Build history of the part. All positions in model axes, mm. A direction names the side the tool comes from. Give positions to 0.01 mm unless a question says otherwise; leave off trailing zeros. Order: outer loops, then holes, each group sorted by start corner. A loop starts at its lowest first (then second) coordinate and runs counter-clockwise, first axis right, second up. Notation, with made-up numbers: (48, 13.5) - (102, 13.5) arc R20 cw to (102, 31.5) - close; hole circle Ø9 at (63, 25.5). An arc over 180 degrees is marked (long way). Use a Markdown table: item, result. Add a question column.
(1) Mould opens along Y. For faces 6 (the face through (18, 2, 2.54)), 7 (the face through (31.772, 12.75, 1.288)), 8 (the face through (27.292, 8.809, 6.332)) say: +Y half, -Y half, draft (parallel to the pull), parting line (faces both ways), or undercut.
(2) Slice it at D-D (z = 11.5). Write the cut outline in (x, y).
(3) Slice it at B-B (y = 10.5). Write the cut outline in (x, z).
(4) Flat gauge pins, fed straight in: pin 1 (1.3 mm diameter, centred on x = 23, z = 4.5, fed in from -Y); pin 2 (5 mm diameter, centred on x = 11, y = 7.5, fed in from +Z); pin 3 (3 mm diameter, centred on x = 11.5, y = 17, fed in from +Z). Where does each tip first touch, or does it go through?
(5) Which spindle directions (+Z, -Z, +X, -X, +Y, -Y) get a long thin tool onto all of the face, cutting with end or side? Do faces 1 (the face through (26, 21, 5.08)), 2 (the face through (7.747, 13, 4)), 3 (the face through (18, 22.86, 4)), 4 (the face through (10, 5, 5.08)), 5 (the face through (26, 5, 5.08)). Say none if no direction does.
(6) Slice it at A-A (x = 33). Write the cut outline in (y, z), then the cut area to 3 significant figures.
(7) Wall check: line 1 (Z direction, x = 2, y = 18); line 2 (Y direction, x = 11.5, z = 3.5); line 3 (Z direction, x = 27.5, y = 8.25). Give the ranges that are in metal, low to high.
(8) Slice it at C-C (x = 16.5). Write the cut outline in (y, z).
from build123d import *

# Parameters (mm, degrees)
SKETCH1_W           = 35.814
SKETCH1_H           = 25.4
BOSS_EXTRUDE1_DEPTH = 2.54
SKETCH2_R           = 1.143
CUT_EXTRUDE1_DEPTH  = 2.54
SKETCH3_W           = 20.32
SKETCH3_H           = 20.32
BOSS_EXTRUDE3_DEPTH = 2.54
SKETCH4_R           = 10.16
BOSS_EXTRUDE4_DEPTH = 2.54
DOME3_FACE_RADIUS   = 10.16
DOME3_HEIGHT        = 7.62


with BuildPart() as part:
    # Sketch1 → Boss-Extrude1 (new body)
    with BuildSketch(Plane.XY):
        with Locations((17.907, 12.7)):
            Rectangle(SKETCH1_W, SKETCH1_H)
    extrude(amount=BOSS_EXTRUDE1_DEPTH)

    # Sketch2 → Cut-Extrude1 (cut)
    with BuildSketch(Plane.XY.offset(2.54)):
        with Locations((2.942, 12.7)):
            Circle(SKETCH2_R)
        with Locations((32.914, 12.7)):
            Circle(SKETCH2_R)
    extrude(amount=-CUT_EXTRUDE1_DEPTH, mode=Mode.SUBTRACT)

    # Sketch3 → Boss-Extrude3 (add)
    with BuildSketch(Plane.XY.offset(2.54)):
        with Locations((17.907, 12.7)):
            Rectangle(SKETCH3_W, SKETCH3_H)
    extrude(amount=BOSS_EXTRUDE3_DEPTH)

    # Sketch4 → Boss-Extrude4 (add)
    with BuildSketch(Plane.XY.offset(5.08)):
        with Locations((17.907, 12.7)):
            Circle(SKETCH4_R)
    extrude(amount=BOSS_EXTRUDE4_DEPTH)

    # Dome3: a dome of height H over a round flat face of radius A is a cap of a sphere of radius (A * A + H * H) / (2 * H)
    dome3_r = (DOME3_FACE_RADIUS * DOME3_FACE_RADIUS + DOME3_HEIGHT * DOME3_HEIGHT) / (2 * DOME3_HEIGHT)
    dome3_base = Plane((17.907, 12.7, 7.62), z_dir=(0, 0, 1))
    with Locations(dome3_base.offset(DOME3_HEIGHT - dome3_r)):
        dome3_ball = Sphere(dome3_r, mode=Mode.PRIVATE)
    add(split(dome3_ball, bisect_by=dome3_base, keep=Keep.TOP, mode=Mode.PRIVATE))


solid = part.part
Solution:
| question | item | result |
|---|---|---|
| 1 | face 6 | draft |
| 1 | face 7 | undercut |
| 1 | face 8 | parting line |
| 2 | outline | circle Ø16.15 at (17.91, 12.7) |
| 3 | outline | (0, 0) - (35.81, 0) - (35.81, 2.54) - (28.07, 2.54) - (28.07, 5.08) - (27.83, 5.08) - (27.83, 7.62) arc R10.35 ccw to (7.99, 7.62) - (7.99, 5.08) - (7.75, 5.08) - (7.75, 2.54) - (0, 2.54) - close |
| 4 | pin 1 | y = 2.54 |
| 4 | pin 2 | z = 13.27 |
| 4 | pin 3 | z = 13.22 |
| 5 | face 1 | +Z, +X, +Y |
| 5 | face 2 | +Z, -X, +Y, -Y |
| 5 | face 3 | +Z, +X, -X, +Y |
| 5 | face 4 | +Z, -X, -Y |
| 5 | face 5 | +Z, +X, -Y |
| 6 | outline | (0, 0) - (11.56, 0) - (11.56, 2.54) - (0, 2.54) - close; (13.84, 0) - (25.4, 0) - (25.4, 2.54) - (13.84, 2.54) - close |
| 6 | area | 58.7 mm2 |
| 7 | line 1 | 0 to 2.54 |
| 7 | line 2 | 2.54 to 22.86 |
| 7 | line 3 | 0 to 5.08 |
| 8 | outline | (0, 0) - (25.4, 0) - (25.4, 2.54) - (22.86, 2.54) - (22.86, 5.08) - (22.76, 5.08) - (22.76, 7.62) arc R10.49 ccw to (2.64, 7.62) - (2.64, 5.08) - (2.54, 5.08) - (2.54, 2.54) - (0, 2.54) - close |
